from build123d import *

# Parameters (mm, degrees)
F0_R     = 101.6
F1_DEPTH = 635
F2_R     = 101.6
F3_DEPTH = 127
F4_DEPTH = 127
F5_SIZE  = 25.4
F6_SIZE  = 5.08


with BuildPart() as f1:
    # F0 (on Top) → F1 (new body)
    with BuildSketch(Plane.XY):
        Circle(F0_R)
    extrude(amount=F1_DEPTH)

    # F2 (on face) → F3 (join)
    with BuildSketch(Plane.XY.offset(635)):
        Polygon((-190.5, 109.9852262806), (-190.5, -109.9852262806), (0, -219.9704525612), (190.5, -109.9852262806), (190.5, 109.9852262806), (0, 219.9704525612), align=None)
        Circle(F2_R, mode=Mode.SUBTRACT)
        Circle(F2_R)
    extrude(amount=F3_DEPTH)

    # F4 (add): a face of the model
    f4_faces = [f1.faces().sort_by_distance(p)[0] for p in [
        (0, 0, 0),
    ]]
    extrude(f4_faces, amount=F4_DEPTH)

    # F5
    f5_edges = [f1.edges().sort_by_distance(p)[0] for p in [
        (-101.6, 0, -127),
    ]]
    chamfer(f5_edges, length=F5_SIZE)

    # F6
    f6_edges = [f1.edges().sort_by_distance(p)[0] for p in [
        (-190.5, 0, 762),
        (-95.25, -164.977839, 762),
        (95.25, -164.977839, 762),
        (190.5, 0, 762),
        (95.25, 164.977839, 762),
        (-95.25, 164.977839, 762),
        (-190.5, 0, 635),
        (-95.25, 164.977839, 635),
        (-95.25, -164.977839, 635),
        (95.25, 164.977839, 635),
        (95.25, -164.977839, 635),
        (190.5, 0, 635),
        (-101.6, 0, 635),
    ]]
    chamfer(f6_edges, length=F6_SIZE)


solid = f1.part
For this review, take the finished solid that the model builds, in its own axes (mm). A direction names the side the tool comes from. Give positions to 0.01 mm unless a question says otherwise; leave off trailing zeros. Order: outer loops, then holes, each group sorted by start corner. A loop starts at its lowest first (then second) coordinate and runs counter-clockwise, first axis right, second up. Notation, with made-up numbers: M 14.5,84 L 31.5,84 A11 ccw 31.5,97 Z; hole C 71,-38.75 d6. An arc over 180 degrees is marked long. Answer in a Markdown table with one row per item. Add a question column.
(1) For pin 1 (4 mm diameter, centred on y = -58.5, z = 429, fed in from +X); pin 2 (3 mm diameter, centred on x = 91.5, y = 83.5, fed in from -Z); pin 3 (3 mm diameter, centred on y = 28, z = 472.5, fed in from -X), all flat-tipped, find the tip position at first contact; note any pin that passes through.
(2) Consider section C-C on z = 330. State the section outline as (x, y) points, and give its area (3 significant figures).
(3) Consider section D-D on x = -131. State the section outline as (y, z) points, and give its area (3 significant figures).
(4) For faces 1 (the face through (-93.917, 165.748, 697.682)), 2 (the face through (-85, -92, 635)), list the 3-axis set-ups (+Z, -Z, +X, -X, +Y, -Y) from which the entire face can be reached by the end or side of a thin tool; tool diameter is ignored.
(5) Consider section B-B on y = 0. State the section outline as (x, z) points, and give its area (3 significant figures).
(6) Consider section A-A on x = 126. State the section outline as (y, z) points.
(7) Wall thickness on probe 1 along Z at (x, y) = (26, 147); probe 2 along Y at (x, z) = (6, 49); probe 3 along X at (y, z) = (-79, -42.5): over which ranges is each line inside the solid? List them lowest first. Write a range as [from, to].
Evaluation:
| question | item | result |
|---|---|---|
| 1 | pin 1 | stops at x = 84.44 |
| 1 | pin 2 | stops at z = 635 |
| 1 | pin 3 | stops at x = -98.08 |
| 2 | outline | C 0,0 d203.2 |
| 2 | area | 32,400 mm^2 |
| 3 | outline | M -144.34,640.08 L -138.47,635 L 138.47,635 L 144.34,640.08 L 144.34,756.92 L 138.47,762 L -138.47,762 L -144.34,756.92 Z |
| 3 | area | 36,600 mm^2 |
| 4 | face 1 | +Z, -Z, -X, +Y |
| 4 | face 2 | -Z |
| 5 | outline | M -190.5,640.08 L -185.42,635 L -106.68,635 L -101.6,629.92 L -101.6,-101.6 L -76.2,-127 L 76.2,-127 L 101.6,-101.6 L 101.6,629.92 L 106.68,635 L 185.42,635 L 190.5,640.08 L 190.5,756.92 L 185.42,762 L -185.42,762 L -190.5,756.92 Z |
| 5 | area | 203,000 mm^2 |
| 6 | outline | M -147.22,640.08 L -141.36,635 L 141.36,635 L 147.22,640.08 L 147.22,756.92 L 141.36,762 L -141.36,762 L -147.22,756.92 Z |
| 7 | probe 1 | z = [635, 762] |
| 7 | probe 2 | y = [-101.42, 101.42] |
| 7 | probe 3 | x = [-63.89, 63.89] |
